```python
from build123d import *

# Parameters (mm, degrees)
F1_DEPTH = 20
F2_R     = 1
F3_W     = 16
F3_H     = 1
F4_DEPTH = 25
F6_DEPTH = 25
F8_DEPTH = 25
F9_SIZE  = 0.5


with BuildPart() as f1:
    # F0 (on Right) → F1 (new body)
    with BuildSketch(Plane.YZ):
        Polygon((-40, 0), (0, 0), (0, 80), (-8, 80), (-8, 8), (-40, 8), align=None)
    extrude(amount=F1_DEPTH)

    # F2
    f2_edges = [f1.edges().sort_by_distance(p)[0] for p in [
        (10, -8, 8),
    ]]
    fillet(f2_edges, radius=F2_R)

    # F3 (on face) → F4 (cut)
    with BuildSketch(Plane.XY.offset(8)):
        with Locations((10, -8.5)):
            Rectangle(F3_W, F3_H)
    extrude(amount=F4_DEPTH, mode=Mode.SUBTRACT)

    # F5 (on face) → F6 (cut)
    with BuildSketch(Plane.XY.offset(8)):
        with BuildLine():
            Line((7, -17), (7, -29))
            ThreePointArc((7, -29), (10, -32), (13, -29))
            Line((13, -29), (13, -17))
            ThreePointArc((13, -17), (10, -14), (7, -17))
        make_face()
    extrude(amount=-F6_DEPTH, mode=Mode.SUBTRACT)

    # F7 (on face) → F8 (cut)
    with BuildSketch(Plane.XZ.offset(8)):
        with BuildLine():
            ThreePointArc((13, 69), (12.12132, 71.12132), (10, 72))
            Line((10, 72), (10, 14))
            ThreePointArc((10, 14), (12.12132, 14.87868), (13, 17))
            Line((13, 17), (13, 69))
        make_face()
        with BuildLine():
            Line((10, 14), (10, 72))
            ThreePointArc((10, 72), (7.87868, 71.12132), (7, 69))
            Line((7, 69), (7, 17))
            ThreePointArc((7, 17), (7.87868, 14.87868), (10, 14))
        make_face()
    extrude(amount=-F8_DEPTH, mode=Mode.SUBTRACT)

    # F9
    f9_edges = [f1.edges().sort_by_distance(p)[0] for p in [
        (10, 0, 80),
        (10, -8, 80),
        (0, -4, 80),
        (20, -4, 80),
        (10, -40, 8),
        (10, -40, 0),
        (0, -40, 4),
        (20, -40, 4),
        (20, -8, 44.5),
        (20, -8.292893, 8.292893),
        (20, -24.5, 8),
        (20, 0, 40),
        (20, -20, 0),
        (0, -8, 44.5),
        (0, -8.292893, 8.292893),
        (0, -24.5, 8),
        (0, 0, 40),
        (0, -20, 0),
        (7, -8, 43),
        (7, 0, 43),
        (7, -23, 0),
        (7, -23, 8),
        (10, 0, 0),
    ]]
    chamfer(f9_edges, length=F9_SIZE)


solid = f1.part
```
Check sheet for the modelled part. Datum: model origin and axes. Units: mm. A direction names the side the tool comes from. Give positions to 0.01 mm unless a question says otherwise; leave off trailing zeros. Loops run counter-clockwise (first coordinate to the right, second up) from the corner with the lowest first, then second, coordinate; pieces in that order, holes last. Notation, with made-up numbers: M 42,73.25 L 55,73.25 A12 ccw 55,88.25 Z; hole C -20.5,72 d10. An arc over 180 degrees is marked long. Answer in a Markdown table with one row per item.
1) Cross-section at C-C (z = 10.5). Enter the section's corners in (x, y), plus the area to 4 significant figures.
Solutions:
| item | result |
|---|---|
| outline | M 0,-7.5 L 0.5,-8 L 19.5,-8 L 20,-7.5 L 20,-0.5 L 19.5,0 L 0.5,0 L 0,-0.5 Z |
| area | 159.5 mm^2 |
2) Thickness scan on line 1 (Y direction, x = 7.5, z = 75); line 2 (Z direction, x = 1, y = -19); line 3 (Z direction, x = 12, y = -7). Record the ranges inside material, lowest first.
Solutions:
| item | result |
|---|---|
| line 1 | y = -8 to 0 |
| line 2 | z = 0 to 8 |
| line 3 | z = 0 to 14.76, 71.24 to 80 |
3) Cross-section at A-A (z = 28.5). Enter the section's corners in (x, y).
Solutions:
| item | result |
|---|---|
| outline | M 0,-7.5 L 0.5,-8 L 6.5,-8 L 7,-7.5 L 7,-0.5 L 6.5,0 L 0.5,0 L 0,-0.5 Z; M 13,-7.5 L 13.5,-8 L 19.5,-8 L 20,-7.5 L 20,-0.5 L 19.5,0 L 13.5,0 L 13,-0.5 Z |
4) Depth check by flat-ended pin: pin 1 (0.5 mm diameter, centred on y = -8.5, z = 8.5, fed in from -X); pin 2 (1.1 mm diameter, centred on y = -8.5, z = 8.5, fed in from +X); pin 3 (4 mm diameter, centred on x = 3.5, y = -8.5, fed in from +Z); pin 4 (5.5 mm diameter, centred on x = 6.5, z = 52, fed in from -Y). Enter the tip coordinate at first touch or a pass-through.
Solutions:
| item | result |
|---|---|
| pin 1 | passes through |
| pin 2 | stops at x = 19.76 |
| pin 3 | stops at z = 80 |
| pin 4 | stops at y = -8 |
5) Tool access check on faces 1 (the face through (10.069, -13.865, 0.365)), 2 (the face through (20, -7, 31)), 3 (the face through (7, -23, 4)), 4 (the face through (14, 0, 39)), 5 (the face through (9.931, -32.135, 7.635)). Record the directions out of +Z, -Z, +X, -X, +Y, -Y that give a thin tool (end or side, any length) a straight path to the whole face; none if there is none.
Solutions:
| item | result |
|---|---|
| face 1 | -Z |
| face 2 | +Z, -Z, +X, +Y, -Y |
| face 3 | +Z, -Z |
| face 4 | +Z, -Z, +X, -X, +Y |
| face 5 | +Z |
6) Cross-section at D-D (y = -33.5). Enter the section's corners in (x, z).
Solutions:
| item | result |
|---|---|
| outline | M 0,0.5 L 0.5,0 L 19.5,0 L 20,0.5 L 20,7.5 L 19.5,8 L 0.5,8 L 0,7.5 Z |
7) Mould release check, pull along Z, two halves, no side actions. Record for faces 6 (the face through (9.931, -32.135, 0.365)), 7 (the face through (0, -7, 31)), 8 (the face through (13, -4, 43)), 9 (the face through (7, -4, 43)): released by +Z, released by -Z, zero draft, split by the parting line, or undercut.
Solutions:
| item | result |
|---|---|
| face 6 | released by -Z |
| face 7 | zero draft |
| face 8 | undercut |
| face 9 | undercut |
8) Cross-section at B-B (y = -6.5). Enter the section's corners in (x, z), plus the area to 3 significant figures.
Solutions:
| item | result |
|---|---|
| outline | M 0,0.5 L 0.5,0 L 19.5,0 L 20,0.5 L 20,79.5 L 19.5,80 L 0.5,80 L 0,79.5 Z; hole M 7,17 A3 ccw 10,14 A3 ccw 13,17 L 13,69 A3 ccw 10,72 A3 ccw 7,69 Z |
| area | 1,260 mm^2 |
